from build123d import *

# Parameters (mm, degrees)
F0_W     = 400
F0_H     = 300
F1_DEPTH = 25
F2_SIZE  = 24.99999


# Not quite as in the source:
# - a fillet or chamfer is up to 0.001 mm smaller than in the source, because OpenCascade refuses the exact size


with BuildPart() as f1:
    # F0 (on Top) → F1 (new body)
    with BuildSketch(Plane.XY):
        Rectangle(F0_W, F0_H)
    extrude(amount=-F1_DEPTH)

    # F2 (size 25 in the source; OpenCascade refuses exactly that, so slightly less here)
    f2_edges = [f1.edges().sort_by_distance(p)[0] for p in [
        (-200, 0, -25),
        (200, 0, -25),
    ]]
    chamfer(f2_edges, length=F2_SIZE)


solid = f1.part
Source: CAD feature listing. Evaluate the final solid. Frame: model axes, mm. Round coordinates to 2 decimals unless told otherwise and drop trailing zeros. Loops run counter-clockwise (first coordinate to the right, second up) from the corner with the lowest first, then second, coordinate; pieces in that order, holes last. Notation, with made-up numbers: (86.5, -11) - (135.5, -11) arc R38 ccw to (135.5, 27) - close; hole circle Ø3 at (47, 85). An arc over 180 degrees is marked (long way). Write item = value, one per line. Start each with the question number.
Item 1: First-contact query: pin 1 Ø4 at (y, z) = (6, -12) entering from -X; pin 2 Ø10 at (y, z) = (-85, -14) entering from -X; pin 3 Ø4 at (y, z) = (86, -19.5) entering from +X. Flat tips, straight axial feed; report the tip coordinate or a pass-through.
Item 2: Section query B-B on z = -13.5. Output: boundary loops of the cut face in (x, y).
Item 3: Material intervals for line 1 (X direction, y = 116.5, z = -24); line 2 (X direction, y = -4.5, z = -11.5); line 3 (Z direction, x = 183, y = -49), sorted ascending.
Results list:
q1.pin_1 = -190
q1.pin_2 = -191
q1.pin_3 = 182.5
q2.outline = (-186.5, -150) - (186.5, -150) - (186.5, 150) - (-186.5, 150) - close
q3.line_1 = -176 to 176
q3.line_2 = -188.5 to 188.5
q3.line_3 = -17 to 0
